from build123d import *

# Parameters (mm, degrees)
BOSS_EXTRUDE2_DEPTH      = 152.4
BOSS_EXTRUDE2_DEPTH_BACK = 152.4
SKETCH3_R                = 25.4
SKETCH3_R_2              = 22.225
SKETCH9_R                = 25.4
SKETCH9_R_2              = 22.225
BOSS_EXTRUDE3_DEPTH      = 88.9
CUT_EXTRUDE2_DEPTH       = 244.959033446
CUT_EXTRUDE2_DEPTH_BACK  = 244.959033446
CUT_EXTRUDE3_DEPTH       = 244.959033566
CUT_EXTRUDE3_DEPTH_BACK  = 244.959033566
SKETCH6_R                = 3.96875
CUT_EXTRUDE4_DEPTH       = 244.959033566
CUT_EXTRUDE4_DEPTH_BACK  = 244.959033566
SKETCH8_R                = 3.96875


with BuildPart() as part:
    # Sketch3 → Boss-Extrude2 (new, two sides: drawn at the far end of the back side and taken through both)
    with BuildSketch(Plane.XY.offset(-BOSS_EXTRUDE2_DEPTH_BACK)):
        Circle(SKETCH3_R)
        Circle(SKETCH3_R_2, mode=Mode.SUBTRACT)
    extrude(amount=BOSS_EXTRUDE2_DEPTH + BOSS_EXTRUDE2_DEPTH_BACK)

    # Sketch9 → Boss-Extrude3 (add)
    with BuildSketch(Plane.XY.offset(152.4)):
        Circle(SKETCH9_R)
        Circle(SKETCH9_R_2, mode=Mode.SUBTRACT)
    extrude(amount=BOSS_EXTRUDE3_DEPTH)

    # Sketch5 → Cut-Extrude2 (cut, two sides: drawn at the far end of the back side and taken through both)
    with BuildSketch(Plane(origin=(0, 0, 0), x_dir=(0, 0, -1), z_dir=(1, 0, 0)).offset(-CUT_EXTRUDE2_DEPTH_BACK)):
        with BuildLine():
            Line((-146.05, 4.7625), (69.85, 4.7625))
            ThreePointArc((69.85, 4.7625), (74.6125, 0), (69.85, -4.7625))
            Line((69.85, -4.7625), (-146.05, -4.7625))
            ThreePointArc((-146.05, -4.7625), (-150.8125, 0), (-146.05, 4.7625))
        make_face()
    extrude(amount=CUT_EXTRUDE2_DEPTH + CUT_EXTRUDE2_DEPTH_BACK, mode=Mode.SUBTRACT)

    # Sketch6 → Cut-Extrude3 (cut, two sides: drawn at the far end of the back side and taken through both)
    with BuildSketch(Plane(origin=(0, 0, 0), x_dir=(0, 0, -1), z_dir=(1, 0, 0)).offset(-CUT_EXTRUDE3_DEPTH_BACK)):
        with Locations((138.641666667, 0)):
            Circle(SKETCH6_R)
    extrude(amount=CUT_EXTRUDE3_DEPTH + CUT_EXTRUDE3_DEPTH_BACK, mode=Mode.SUBTRACT)

    # Sketch8 → Cut-Extrude4 (cut, two sides: drawn at the far end of the back side and taken through both)
    with BuildSketch(Plane(origin=(0, 0, 0), x_dir=(1, 0, 0), z_dir=(0, 1, 0)).offset(-CUT_EXTRUDE4_DEPTH_BACK)):
        with Locations(Location((0, 124.883333333, 0), (0, 0, 270))):
            Circle(SKETCH8_R)
    extrude(amount=CUT_EXTRUDE4_DEPTH + CUT_EXTRUDE4_DEPTH_BACK, mode=Mode.SUBTRACT)


solid = part.part
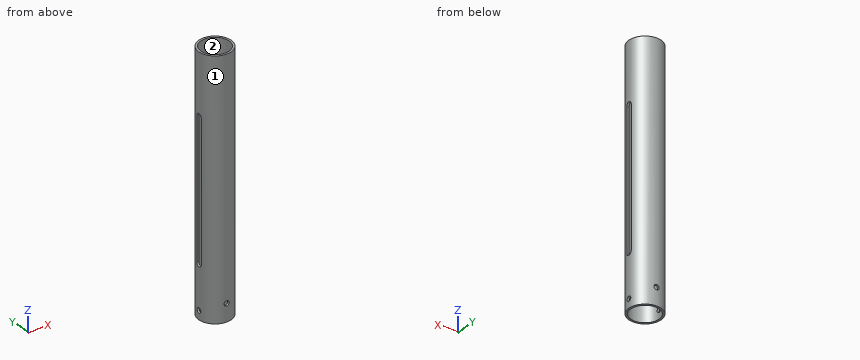
The listing builds one solid part. Answer for the finished solid, in the listing's coordinates (mm). Face numbers are marked on the shaded views. Round coordinates to 2 decimals unless told otherwise and drop trailing zeros. Write each loop counter-clockwise with the first axis right and the second up, starting at its lowest first coordinate (ties: lowest second). Pieces come first, ordered by that corner, then holes. Notation, with made-up numbers: M 28,36.25 L 86,36.25 A9 ccw 86,48.25 Z; hole C 65.25,84 d8. An arc over 180 degrees is marked long. Write each question's results on one line, items separated by ' | '. Start each with the question number.
(1) Each of these flat-tipped pins is pushed along its axis until it touches: P1, Ø2.5, axis at x = -23.5, z = 57, coming from the -Y side; P2, Ø3.5, axis at x = 23.5, z = 41, coming from the +Y side; P3, Ø1, axis at y = 9, z = 97.5, coming from the -X side. Where does it stop, or does it pass through?
(2) Determine the mould class of the marked faces 1 and 2 for opening direction X: +X half, -X half, draft (parallel to the pull), parting line (faces both ways), or undercut.
(3) The part is cut by section A-A, the plane x = 0. Write down the section's boundary in (y, z) (3 decimals), and give its area (3 significant figures).
(4) The part is cut by section C-C, the plane y = -15. Write down the section's boundary in (x, z).
(5) Find the intervals of material crossed by line 1 (Z direction, x = 24, y = 0); line 2 (Y direction, x = -1, z = -93.5); line 3 (X direction, y = 5, z = -1), in increasing order.
Worked answers:
1) P1: stops at y = -12.25 | P2: stops at y = 13.12 | P3: stops at x = -23.94
2) face 1: parting line | face 2: undercut
3) outline: M -25.4,-152.4 L -22.225,-152.4 L -22.225,-128.852 L -25.4,-128.852 Z; M -25.4,-120.915 L -22.225,-120.915 L -22.225,241.3 L -25.4,241.3 Z; M 22.225,-152.4 L 25.4,-152.4 L 25.4,-128.852 L 22.225,-128.852 Z; M 22.225,-120.915 L 25.4,-120.915 L 25.4,241.3 L 22.225,241.3 Z | area: 2,450 mm²
4) outline: M -20.5,-152.4 L -16.4,-152.4 L -16.4,241.3 L -20.5,241.3 Z; M 16.4,-152.4 L 20.5,-152.4 L 20.5,241.3 L 16.4,241.3 Z
5) line 1: z = -152.4 to -142.61, -134.67 to -74.61, 150.81 to 241.3 | line 2: y = -25.38 to -22.2, 22.2 to 25.38 | line 3: x = -24.9 to -21.66, 21.66 to 24.9
